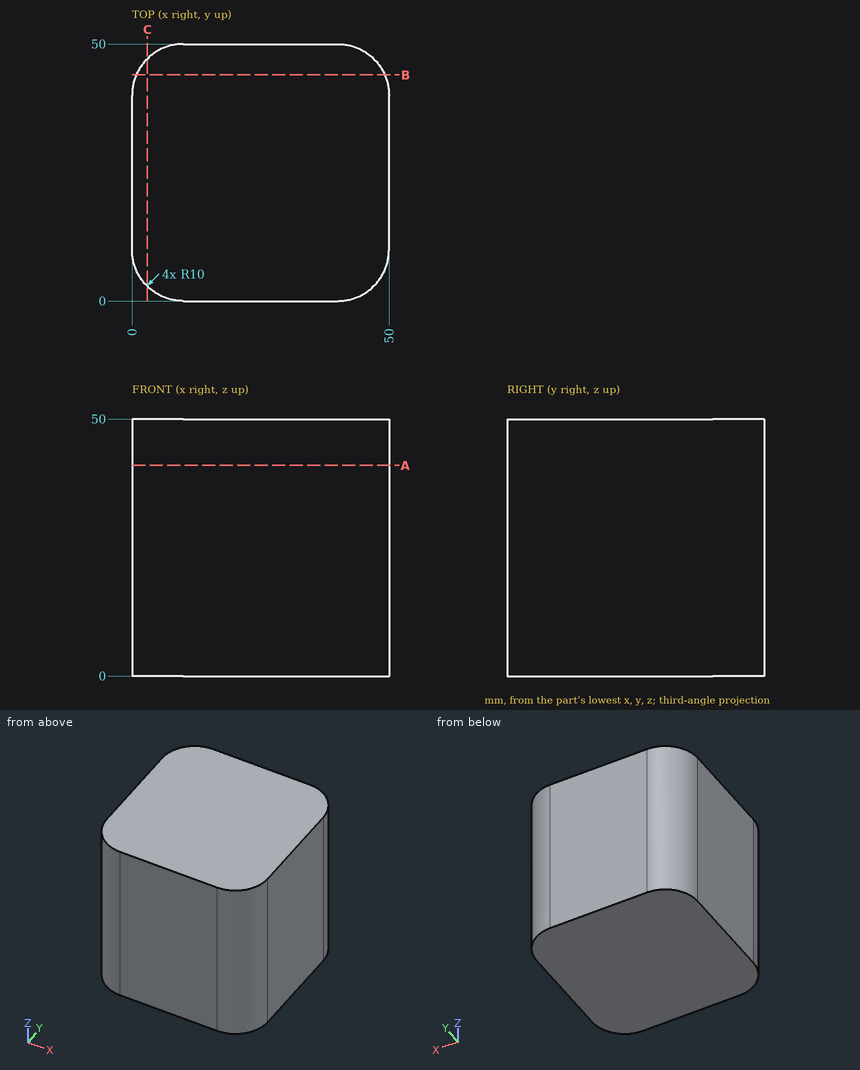
Can you work these out from the drawing? Everything is in mm from the part's minimum corner. Coordinates: 2 decimals unless noted, no trailing zeros. Loops run counter-clockwise (first coordinate to the right, second up) from the corner with the lowest first, then second, coordinate; pieces in that order, holes last.
1. Imagine slicing it at A-A, the plane z = 41. Please give me the cut outline in (x, y), and give its area (3 significant figures).
2. Imagine slicing it at C-C, the plane x = 3. Please give me the cut outline in (y, z).
3. For P1, Ø8, axis at y = 40.5, z = 27.5, coming from the -X side, with a flat end and sliding along its axis, tell me the tip position at first contact or that it passes through.
4. Imagine slicing it at B-B, the plane y = 44. Please give me the cut outline in (x, z), and give its area (3 significant figures).
5. I need wall thicknesses on L1, parallel to Y at x = 42, z = 10; L2, parallel to X at y = 7.5, z = 27; L3, parallel to Y at x = 4, z = 16. Which ranges of each line are inside material? Lowest first, please.
Taken from the geometry:
1. outline: (0, 10) arc R10 ccw to (10, 0) - (40, 0) arc R10 ccw to (50, 10) - (50, 40) arc R10 ccw to (40, 50) - (10, 50) arc R10 ccw to (0, 40) - close
1. area: 2,410 mm2
2. outline: (2.86, 0) - (47.14, 0) - (47.14, 50) - (2.86, 50) - close
3. P1: stops at x = 0
4. outline: (0.83, 0) - (49.17, 0) - (49.17, 50) - (0.83, 50) - close
4. area: 2,420 mm2
5. L1: y = 0.2 to 49.8
5. L2: x = 0.32 to 49.68
5. L3: y = 2 to 48
